For this review, take the finished solid that the model builds, in its own axes (mm). Coordinates: 2 decimals unless noted, no trailing zeros. Loops run counter-clockwise (first coordinate to the right, second up) from the corner with the lowest first, then second, coordinate; pieces in that order, holes last. Notation, with made-up numbers: (12.25, 20) - (45.25, 20) arc R32 cw to (45.25, 56) - close; hole circle Ø7 at (30, -12). An arc over 180 degrees is marked (long way). Answer as a JSON object with one key per item and string values. Group by question number.
Item 1: We need section B-B (z = 16.25). Give the boundary of the cut face in (x, y).
Item 2: We need section A-A (y = 196). Give the boundary of the cut face in (x, z), then the cut area to 3 significant figures.
Item 3: Clearance check with flat-ended pins moving along their axes: pin 1 (1.5 mm diameter, centred on x = -201, y = 247.5, fed in from +Z); pin 2 (3.5 mm diameter, centred on x = 35.71, z = 10, fed in from +Y). State where each tip first meets the part, or that it passes through.
Item 4: Mouldability with a two-part tool opening along X and no side actions: class faces 1 (the flat face through (-275, 5, 10)), 2 (the flat face through (275, -5, 10)), 3 (the flat face through (-3, 4, 7)), 4 (the flat face through (-4, -337.5, 10)) as released by +X, released by -X, zero draft, split by the parting line, or undercut.
Item 5: We need section C-C (x = -200). Give the boundary of the cut face in (y, z).
Item 6: To check wall thickness, follow line 1 (X direction, y = 331, z = 10); line 2 (Y direction, x = 130.5, z = 9); line 3 (Z direction, x = -26.5, y = 210.5). State the ranges of each line that lie inside material, in increasing order.
Autodesk Inventor part; units mm, degrees
ref_plane "YZ Plane" through (0, 0, 0) normal (1, 0, 0) x (0, 1, 0)
ref_plane "XZ Plane" through (0, 0, 0) normal (0, 1, 0) x (-1, 0, 0)
ref_plane "XY Plane" through (0, 0, 0) normal (0, 0, 1) x (1, 0, 0)
sketch "Sketch1" plane through (0, 0, 0) normal (0, 0, 1) x (1, 0, 0)
  line L0 (-275, -337.5) -> (275, -337.5)
  line L1 (275, -337.5) -> (275, 337.5)
  line L2 (275, 337.5) -> (-275, 337.5)
  line L3 (-275, 337.5) -> (-275, -337.5)
  line L4 (-275, -337.5) -> (275, 337.5) construction
  line L5 (275, -337.5) -> (-275, 337.5) construction
  point P0 (0, 0)
  dimension "d0" = 550
  dimension "d1" = 675
extrude "Extrusion1" add sketch "Sketch1" along normal blind 20
sketch "Sketch2" plane through (0, 0, 20) normal (0, 0, 1) x (1, 0, 0)
  line L0 (-250, -312.5) -> (250, -312.5)
  line L1 (250, -312.5) -> (250, 312.5)
  line L2 (250, 312.5) -> (-250, 312.5)
  line L3 (-250, 312.5) -> (-250, -312.5)
  line L4 (-250, -312.5) -> (250, 312.5) construction
  line L5 (250, -312.5) -> (-250, 312.5) construction
  point P0 (0, 0)
  dimension "d4" = 500
  dimension "d5" = 625
extrude "Extrusion2" cut sketch "Sketch2" against normal blind 13
sketch "Sketch3" plane through (-275, 337.5, 0) normal (0, 1, 0) x (1, 0, 0)
  line L0 (550, 0) -> (550, -20)
  line L1 (0, 0) -> (0, -20)
  line L2 (0, 0) -> (0, -20)
  line L3 (0, -10) -> (230.6764, -10)
  line L4 (525, -7) -> (25, -7)
  line L5 (0, -10) -> (230.6764, -10) construction
  line L6 (319.3236, 0) -> (230.6764, 0)
  line L7 (230.6764, 0) -> (230.6764, -20)
  line L8 (230.6764, -20) -> (319.3236, -20)
  line L9 (319.3236, -20) -> (319.3236, 0)
  line L10 (319.3236, 0) -> (230.6764, -20) construction
  line L11 (230.6764, 0) -> (319.3236, -20) construction
  circle A0 centre (239.2871, -10) radius 2.1828
  line L12 (275, 0) -> (275, -20)
  circle A1 centre (310.7129, -10) radius 2.1828
  point P0 (275, -10)
  dimension "d8" = 550
  dimension "d9" = 230.6764
  dimension "d10" = 0
  dimension "d11" = 4.3656
  dimension "d12" = 8.6106
extrude "Extrusion3" cut sketch "Sketch3" against normal blind 15 contours A0 | A1
properties part number "WoodFrame"
Check sheet entries:
{
 "1": {"outline": "(-275, -337.5) - (275, -337.5) - (275, 337.5) - (-275, 337.5) - close; hole (-250, -312.5) - (250, -312.5) - (250, 312.5) - (-250, 312.5) - close"},
 "2": {"outline": "(-275, 0) - (275, 0) - (275, 20) - (250, 20) - (250, 7) - (-250, 7) - (-250, 20) - (-275, 20) - close", "area": "4,500 mm2"},
 "3": {"pin 1": "stops at z = 7", "pin 2": "stops at y = 322.5"},
 "4": {"face 1": "released by -X", "face 2": "released by +X", "face 3": "undercut", "face 4": "zero draft"},
 "5": {"outline": "(-337.5, 0) - (337.5, 0) - (337.5, 20) - (312.5, 20) - (312.5, 7) - (-312.5, 7) - (-312.5, 20) - (-337.5, 20) - close"},
 "6": {"line 1": "x = -275 to -37.9, -33.53 to 33.53, 37.9 to 275", "line 2": "y = -337.5 to -312.5, 312.5 to 337.5", "line 3": "z = 0 to 7"}
}
